Print and shaded views of the part. All mm, measured from the part's lowest x, y and z. A direction names the side the tool comes from. Give positions to 0.01 mm unless a question says otherwise; leave off trailing zeros. Loops run counter-clockwise (first coordinate to the right, second up) from the corner with the lowest first, then second, coordinate; pieces in that order, holes last. Notation, with made-up numbers: (62, -28) -> (94, -28) arc R10 ccw to (94, -9) -> close; hole circle Ø7 at (41.5, -36.75). An arc over 180 degrees is marked (long way). Answer as a JSON object with one key per item and string values. Group by question number.
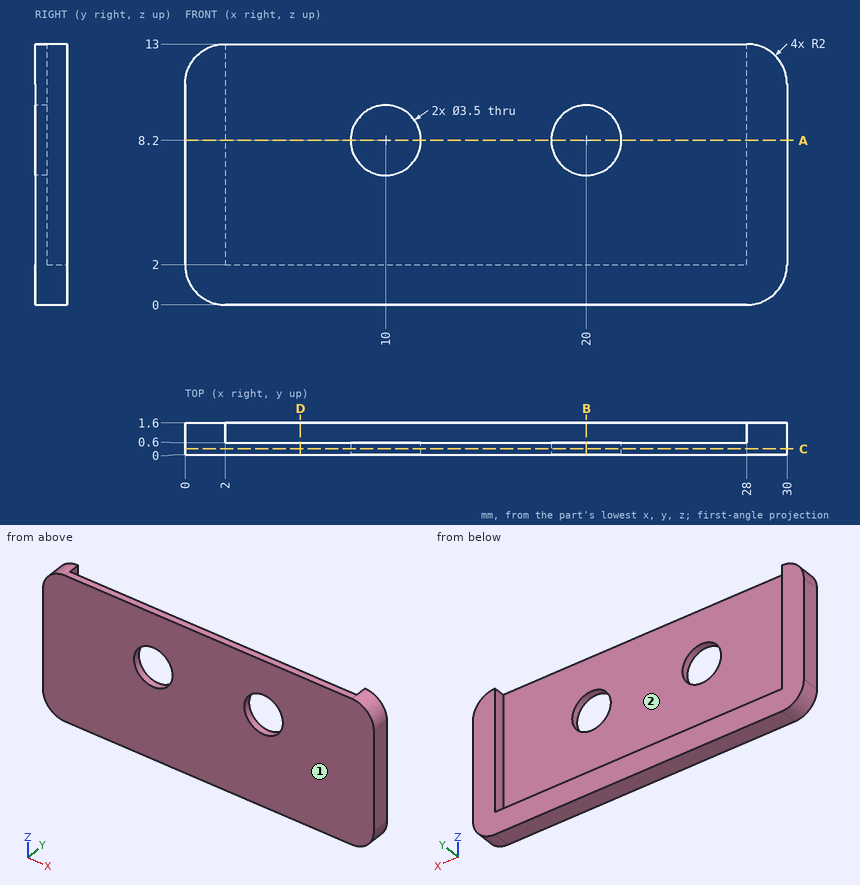
(1) Saw through at C-C on y = 0.3. List the corners of the cut face in (x, z).
(2) Pin check, flat tips, straight feed: pin 1 (4 mm diameter, centred on x = 10, z = 8.2, fed in from +Y); pin 2 (2 mm diameter, centred on x = 20, z = 8.2, fed in from +Y); pin 3 (0.5 mm diameter, centred on x = 12.5, y = 1, fed in from +Z). Stop position of each tip, or through.
(3) Saw through at B-B on x = 20. List the corners of the cut face in (y, z), plus the area to 3 significant figures.
(4) Saw through at A-A on z = 8.2. List the corners of the cut face in (x, y).
(5) Saw through at D-D on x = 5.75. List the corners of the cut face in (y, z), plus the area to 3 significant figures.
(6) Probe line 1 along X through (y, z) = (1.3, 10.25); line 2 along Z through (x, y) = (20, 0.45); line 3 along Y through (x, z) = (6.75, 10.5). List the from-to ranges inside material, lowest first. Write a range as [from, to].
(7) 3-axis set-ups, long thin cutter, end or side, ignore diameter. For the marked faces 1 and 2: which of +Z, -Z, +X, -X, +Y, -Y reach the whole face in a straight line?
Calculated:
{
 "1": {"outline": "(0, 2) arc R2 ccw to (2, 0) -> (28, 0) arc R2 ccw to (30, 2) -> (30, 11) arc R2 ccw to (28, 13) -> (2, 13) arc R2 ccw to (0, 11) -> close; hole circle Ø3.5 at (10, 8.2); hole circle Ø3.5 at (20, 8.2)"},
 "2": {"pin 1": "stops at y = 0.6", "pin 2": "passes through", "pin 3": "stops at z = 2"},
 "3": {"outline": "(0, 0) -> (1.6, 0) -> (1.6, 2) -> (0.6, 2) -> (0.6, 6.45) -> (0, 6.45) -> close; (0, 9.95) -> (0.6, 9.95) -> (0.6, 13) -> (0, 13) -> close", "area": "7.70 mm^2"},
 "4": {"outline": "(0, 0) -> (8.25, 0) -> (8.25, 0.6) -> (2, 0.6) -> (2, 1.6) -> (0, 1.6) -> close; (11.75, 0) -> (18.25, 0) -> (18.25, 0.6) -> (11.75, 0.6) -> close; (21.75, 0) -> (30, 0) -> (30, 1.6) -> (28, 1.6) -> (28, 0.6) -> (21.75, 0.6) -> close"},
 "5": {"outline": "(0, 0) -> (1.6, 0) -> (1.6, 2) -> (0.6, 2) -> (0.6, 13) -> (0, 13) -> close", "area": "9.80 mm^2"},
 "6": {"line 1": "x = [0, 2], [28, 30]", "line 2": "z = [0, 6.45], [9.95, 13]", "line 3": "y = [0, 0.6]"},
 "7": {"face 1": "+Z, -Z, +X, -X, -Y", "face 2": "+Z, +Y"}
}
